Model file for the job. Use its own axes, mm. A direction names the side the tool comes from. Round coordinates to 2 decimals unless told otherwise and drop trailing zeros. Order: outer loops, then holes, each group sorted by start corner. A loop starts at its lowest first (then second) coordinate and runs counter-clockwise, first axis right, second up. Notation, with made-up numbers: (68.25, 62.25) - (120.25, 62.25) arc R36 cw to (120.25, 99.25) - close; hole circle Ø10 at (-12.5, 85.25). An arc over 180 degrees is marked (long way). Write item = value, one per line.
```python
from build123d import *

# Parameters (mm, degrees)
F0_W     = 40
F0_H     = 40
F0_H_2   = 1000
F1_DEPTH = 3
F2_W     = 2000
F2_H     = 1080
F2_W_2   = 1994
F2_H_2   = 1074
F2_W_3   = 1926
F2_H_3   = 1006
F2_W_4   = 40
F2_H_4   = 1000
F2_W_5   = 34
F2_H_5   = 994
F3_DEPTH = 34
F4_W     = 2000
F4_H     = 1080
F4_W_2   = 40
F4_H_2   = 1000
F4_W_3   = 34
F4_H_3   = 994
F5_DEPTH = 3


with BuildPart() as f1:
    # F0 (on Top) → F1 (new body)
    with BuildSketch(Plane.XY):
        with Locations((0, 520)):
            Rectangle(F0_W, F0_H)
        Polygon((-20, 500), (-20, 540), (-1000, 540), (-1000, -540), (-20, -540), (-20, -500), (-960, -500), (-960, 500), align=None)
        Polygon((1000, 540), (20, 540), (20, 500), (960, 500), (960, -500), (20, -500), (20, -540), (1000, -540), align=None)
        with Locations((0, -520)):
            Rectangle(F0_W, F0_H)
        Rectangle(F0_W, F0_H_2)
    extrude(amount=F1_DEPTH)

    # F2 (on face) → F3 (join)
    with BuildSketch(Plane.XY.offset(3)):
        Rectangle(F2_W, F2_H)
        Rectangle(F2_W_2, F2_H_2, mode=Mode.SUBTRACT)
        Rectangle(F2_W_3, F2_H_3)
        Polygon((-20, 500), (20, 500), (960, 500), (960, -500), (20, -500), (-20, -500), (-960, -500), (-960, 500), align=None, mode=Mode.SUBTRACT)
        Rectangle(F2_W_4, F2_H_4)
        Rectangle(F2_W_5, F2_H_5, mode=Mode.SUBTRACT)
    extrude(amount=F3_DEPTH)

    # F4 (on face) → F5 (join)
    with BuildSketch(Plane.XY.offset(37)):
        Rectangle(F4_W, F4_H)
        Polygon((20, 500), (960, 500), (960, -500), (20, -500), (-20, -500), (-960, -500), (-960, 500), (-20, 500), align=None, mode=Mode.SUBTRACT)
        Rectangle(F4_W_2, F4_H_2)
        Rectangle(F4_W_3, F4_H_3, mode=Mode.SUBTRACT)
        Rectangle(F4_W_3, F4_H_3)
    extrude(amount=F5_DEPTH)


solid = f1.part
```
1) Cut at A-A (x = 255). Write the cut outline in (y, z).
Conclusion:
outline = (-540, 0) - (-500, 0) - (-500, 40) - (-540, 40) - close; (500, 0) - (540, 0) - (540, 40) - (500, 40) - close; hole (-537, 3) - (-503, 3) - (-503, 37) - (-537, 37) - close; hole (503, 3) - (537, 3) - (537, 37) - (503, 37) - close
2) Wall check: line 1 along X through (y, z) = (448, 13.5); line 2 along X through (y, z) = (-228, 2); line 3 along Y through (x, z) = (-497, 14.5). Give the ranges that are in metal, low to high.
Conclusion:
line_1 = -1000 to -997, -963 to -960, -20 to -17, 17 to 20, 960 to 963, 997 to 1000
line_2 = -1000 to -960, -20 to 20, 960 to 1000
line_3 = -540 to -537, -503 to -500, 500 to 503, 537 to 540
3) 3-axis set-ups, long thin cutter, end or side, ignore diameter. For faces 4 (the face through (-300, -515, 37)), 5 (the face through (1000, -8, 20)), 6 (the face through (-20, -7, 20)): which of +Z, -Z, +X, -X, +Y, -Y reach the whole face in a straight line?
Conclusion:
face_4 = none
face_5 = +Z, -Z, +X, +Y, -Y
face_6 = +Z, -Z
4) Cut at C-C (z = 24). Write the cut outline in (x, y).
Conclusion:
outline = (-1000, -540) - (1000, -540) - (1000, 540) - (-1000, 540) - close; (-963, -503) - (963, -503) - (963, 503) - (-963, 503) - close; hole (-997, -537) - (997, -537) - (997, 537) - (-997, 537) - close; hole (-960, -500) - (-20, -500) - (-20, 500) - (-960, 500) - close; hole (-17, -497) - (17, -497) - (17, 497) - (-17, 497) - close; hole (20, -500) - (960, -500) - (960, 500) - (20, 500) - close
5) Mould opens along Z. For faces 1 (the face through (-5, 3, 40)), 2 (the face through (-300, -515, 3)), 3 (the face through (20, -7, 20)) say: +Z half, -Z half, draft (parallel to the pull), parting line (faces both ways), or undercut.
Conclusion:
face_1 = +Z half
face_2 = undercut
face_3 = draft
6) Cut at B-B (y = -85.5). Write the cut outline in (x, z), and give its area (3 significant figures).
Conclusion:
outline = (-1000, 0) - (-960, 0) - (-960, 40) - (-1000, 40) - close; (-20, 0) - (20, 0) - (20, 40) - (-20, 40) - close; (960, 0) - (1000, 0) - (1000, 40) - (960, 40) - close; hole (-997, 3) - (-963, 3) - (-963, 37) - (-997, 37) - close; hole (-17, 3) - (17, 3) - (17, 37) - (-17, 37) - close; hole (963, 3) - (997, 3) - (997, 37) - (963, 37) - close
area = 1,330 mm^2
